from build123d import *

# Parameters (mm, degrees)
F0_R     = 4.445
F1_DEPTH = 31.75
F3_DEPTH = 31.751


with BuildPart() as f1:
    # F0 (on Top) → F1 (new body)
    with BuildSketch(Plane.XY):
        with BuildLine():
            ThreePointArc((8.0645, 0), (5.702463, 5.702463), (0, 8.0645))
            ThreePointArc((0, 8.0645), (-5.702463, 5.702463), (-8.0645, 0))
            Line((-8.0645, 0), (-8.0645, -13.342164))
            Line((-8.0645, -13.342164), (-14.986, -22.517859))
            Line((-14.986, -22.517859), (0, -22.517859))
            Line((0, -22.517859), (14.986, -22.517859))
            Line((14.986, -22.517859), (8.0645, -13.342164))
            Line((8.0645, -13.342164), (8.0645, 0))
        make_face()
        with BuildLine():
            Line((0, -13.342164), (-5.207, -13.342164))
            Line((-5.207, -13.342164), (-5.207, -5.388154))
            ThreePointArc((-5.207, -5.388154), (-2.808168, -6.946887), (0, -7.493))
            ThreePointArc((0, -7.493), (2.808168, -6.946887), (5.207, -5.388154))
            Line((5.207, -5.388154), (5.207, -13.342164))
            Line((5.207, -13.342164), (0, -13.342164))
        make_face(mode=Mode.SUBTRACT)
        Circle(F0_R, mode=Mode.SUBTRACT)
    extrude(amount=F1_DEPTH)

    # F2 (on face) → F3 (cut, through all)
    with BuildSketch(Plane.XY.offset(31.75)):
        Polygon((5.207, -15.420636), (-5.2451, -15.420636), (-10.598746, -22.517859), (10.560646, -22.517859), align=None)
    extrude(amount=-F3_DEPTH, mode=Mode.SUBTRACT)


solid = f1.part
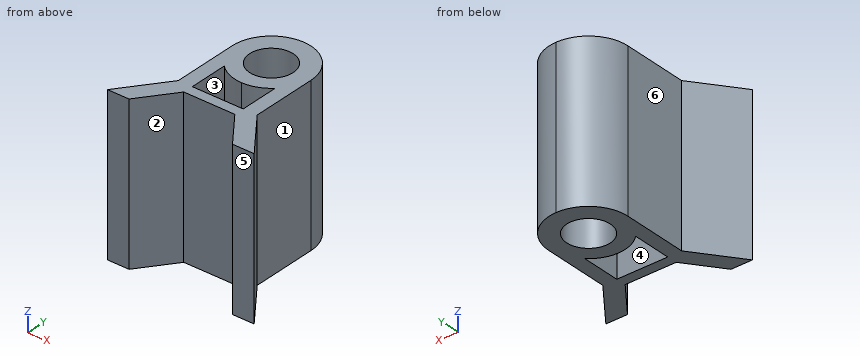
Verification items for the finished model (mm, model axes). Face numbers are marked on the shaded views. A direction names the side the tool comes from. Give positions to 0.01 mm unless a question says otherwise; leave off trailing zeros. Loops run counter-clockwise (first coordinate to the right, second up) from the corner with the lowest first, then second, coordinate; pieces in that order, holes last.
1) Sectioned sample at A-A, the plane y = -10.5. Enter the section's corners in (x, z).
2) Sectioned sample at B-B, the plane z = 11.5. Enter the section's corners in (x, y) (1 decimal), then the cut area to 3 significant figures.
3) Sectioned sample at C-C, the plane x = 12. Enter the section's corners in (y, z).
4) Set-up check for the marked faces 1, 2 and 3: record each of +Z, -Z, +X, -X, +Y, -Y from which the full face is reachable in a straight line by a thin tool's end or side.
5) Draft check along X on the marked faces 4, 5 and 6. Enter one of: pulls with the +X half, pulls with the -X half, needs draft (parallel to the pull), parting line crosses it, or undercut.
6) Thickness scan on line 1 along Y through (x, z) = (0, 17) (1 decimal); line 2 along Y through (x, z) = (0.75, 9); line 3 along X through (y, z) = (-11, 7). Record the ranges inside material, lowest first.
7) Depth check by flat-ended pin: pin 1 Ø4 at (y, z) = (-9.5, 12) entering from -X; pin 2 Ø3 at (x, z) = (0, 22) entering from -Y; pin 3 Ø2 at (x, y) = (3, 1) entering from +Z; pin 4 Ø6.5 at (y, z) = (-9, 18.5) entering from +X. Enter the tip coordinate at first touch or a pass-through.
Answers:
1. outline: (-8.06, 0) - (-5.21, 0) - (-5.21, 31.75) - (-8.06, 31.75) - close; (5.21, 0) - (8.06, 0) - (8.06, 31.75) - (5.21, 31.75) - close
2. outline: (-15, -22.5) - (-10.6, -22.5) - (-5.2, -15.4) - (5.2, -15.4) - (10.6, -22.5) - (15, -22.5) - (8.1, -13.3) - (8.1, 0) arc R8.1 ccw to (0, 8.1) arc R8.1 ccw to (-8.1, 0) - (-8.1, -13.3) - close; hole (-5.2, -13.3) - (5.2, -13.3) - (5.2, -5.4) arc R7.5 cw to (0, -7.5) arc R7.5 cw to (-5.2, -5.4) - close; hole circle Ø8.9 at (0, 0)
2. area: 287 mm2
3. outline: (-22.52, 0) - (-18.56, 0) - (-18.56, 31.75) - (-22.52, 31.75) - close
4. face 1: +Z, -Z, +X, +Y
4. face 2: +Z, -Z, -Y
4. face 3: +Z, -Z
5. face 4: undercut
5. face 5: needs draft
5. face 6: pulls with the -X half
6. line 1: y = -15.4 to -13.3, -7.5 to -4.4, 4.4 to 8.1
6. line 2: y = -15.42 to -13.34, -7.46 to -4.38, 4.38 to 8.03
6. line 3: x = -8.06 to -5.21, 5.21 to 8.06
7. pin 1: stops at x = -8.06
7. pin 2: stops at y = -15.42
7. pin 3: passes through
7. pin 4: stops at x = 8.06
